Geometry: final body of the model. Coordinates: model frame, mm. A direction names the side the tool comes from. Give positions to 0.01 mm unless a question says otherwise; leave off trailing zeros. Loops run counter-clockwise (first coordinate to the right, second up) from the corner with the lowest first, then second, coordinate; pieces in that order, holes last. Notation, with made-up numbers: (59, 40) - (114, 40) arc R22 ccw to (114, 68) - close; hole circle Ø9 at (23, 13.5). An arc over 180 degrees is marked (long way). Answer in a Markdown table with one row per item.
from build123d import *

# Parameters (mm, degrees)
F0_W      = 76.2
F0_H      = 20.32
F0_R      = 1.905
F1_DEPTH  = 1.524
F2_W      = 50.292
F2_H      = 19.05
F3_DEPTH  = 8.128
F4_W      = 53.467
F4_H      = 35.814
F4_R      = 1.905
F5_DEPTH  = 1.6002
F6_W      = 25.4
F6_H      = 10.16
F7_DEPTH  = 8.128
F8_R      = 1.15
F9_DEPTH  = 3
F11_DEPTH = 3.6
F12_W     = 25
F12_H     = 5
F13_DEPTH = 1.6


with BuildPart() as f1:
    # F0 (on Top) → F1 (new body)
    with BuildSketch(Plane.XY):
        Rectangle(F0_W, F0_H)
        with Locations((-33.02, 0)):
            Circle(F0_R, mode=Mode.SUBTRACT)
        with Locations((33.02, 0)):
            Circle(F0_R, mode=Mode.SUBTRACT)
    extrude(amount=F1_DEPTH)

    # F2 (on face) → F3 (join)
    with BuildSketch(Plane.XY.offset(1.524)):
        Rectangle(F2_W, F2_H)
    extrude(amount=F3_DEPTH)


with BuildPart() as f5:
    # F4 (on Top) → F5 (new body)
    with BuildSketch(Plane.XY):
        with Locations((55.63927, 42.330817)):
            Rectangle(F4_W, F4_H)
        with Locations((33.98577, 40.933817)):
            Circle(F4_R, mode=Mode.SUBTRACT)
        with Locations((72.08577, 40.933817)):
            Circle(F4_R, mode=Mode.SUBTRACT)
    extrude(amount=F5_DEPTH)

    # F6 (on face) → F7 (join)
    with BuildSketch(Plane.XY.offset(1.6002)):
        with Locations((53.03577, 40.933817)):
            Rectangle(F6_W, F6_H)
    extrude(amount=F7_DEPTH)


with BuildPart() as f9:
    # F8 (on Top) → F9 (new body)
    with BuildSketch(Plane.XY):
        with BuildLine():
            ThreePointArc((34.542687, -63.528296), (35.27492, -65.296063), (37.042687, -66.028296))
            Line((37.042687, -66.028296), (97.042687, -66.028296))
            ThreePointArc((97.042687, -66.028296), (98.810454, -65.296063), (99.542687, -63.528296))
            Line((99.542687, -63.528296), (99.542687, -4.528296))
            ThreePointArc((99.542687, -4.528296), (98.810454, -2.760529), (97.042687, -2.028296))
            Line((97.042687, -2.028296), (37.042687, -2.028296))
            ThreePointArc((37.042687, -2.028296), (35.27492, -2.760529), (34.542687, -4.528296))
            Line((34.542687, -4.528296), (34.542687, -63.528296))
        make_face()
        with Locations((37.042687, -63.528296)):
            Circle(F8_R, mode=Mode.SUBTRACT)
        with Locations((97.042687, -63.528296)):
            Circle(F8_R, mode=Mode.SUBTRACT)
        with Locations((37.042687, -4.528296)):
            Circle(F8_R, mode=Mode.SUBTRACT)
        with Locations((97.042687, -4.528296)):
            Circle(F8_R, mode=Mode.SUBTRACT)
    extrude(amount=F9_DEPTH)

    # F10 (on face) → F11 (join)
    with BuildSketch(Plane.XY.offset(3)):
        with BuildLine():
            Line((93.042687, -5.528296), (41.042687, -5.528296))
            ThreePointArc((41.042687, -5.528296), (38.21426, -6.699869), (37.042687, -9.528296))
            Line((37.042687, -9.528296), (37.042687, -58.528296))
            ThreePointArc((37.042687, -58.528296), (38.21426, -61.356723), (41.042687, -62.528296))
            Line((41.042687, -62.528296), (93.042687, -62.528296))
            ThreePointArc((93.042687, -62.528296), (95.871114, -61.356723), (97.042687, -58.528296))
            Line((97.042687, -58.528296), (97.042687, -9.528296))
            ThreePointArc((97.042687, -9.528296), (95.871114, -6.699869), (93.042687, -5.528296))
        make_face()
    extrude(amount=F11_DEPTH)

    # F12 (on face) → F13 (join)
    with BuildSketch(Plane(origin=(0, 0, 0), x_dir=(1, 0, 0), z_dir=(0, 0, -1))):
        with Locations((54.542687, 68.528296)):
            Rectangle(F12_W, F12_H)
        with Locations((79.542687, 68.528296)):
            Rectangle(F12_W, F12_H)
    extrude(amount=-F13_DEPTH)


solid = f1.part
Q1. Cut plane A-A (y = 0). Output: boundary loops of the cut face in (x, z) (3 decimals).
Check values:
| item | result |
|---|---|
| outline | (-38.1, 0) - (-34.925, 0) - (-34.925, 1.524) - (-38.1, 1.524) - close; (-31.115, 0) - (31.115, 0) - (31.115, 1.524) - (25.146, 1.524) - (25.146, 9.652) - (-25.146, 9.652) - (-25.146, 1.524) - (-31.115, 1.524) - close; (34.925, 0) - (38.1, 0) - (38.1, 1.524) - (34.925, 1.524) - close |
Q2. Draft query along Y for faces 4 (the flat face through (0, 9.525, 6)), 5 (the flat face through (-1, -10.16, 1)), 6 (the flat face through (-25.146, 0, 6)), 7 (the cylindrical face through (31.117, 0.084, 0.751)). Return one class per face: pulls with the +Y half, pulls with the -Y half, needs draft (parallel to the pull), parting line crosses it, or undercut.
Check values:
| item | result |
|---|---|
| face 4 | pulls with the +Y half |
| face 5 | pulls with the -Y half |
| face 6 | needs draft |
| face 7 | undercut |
Q3. Cut plane D-D (x = 5.5). Output: boundary loops of the cut face in (y, z) (3 decimals), and give its area (3 significant figures).
Check values:
| item | result |
|---|---|
| outline | (-10.16, 0) - (10.16, 0) - (10.16, 1.524) - (9.525, 1.524) - (9.525, 9.652) - (-9.525, 9.652) - (-9.525, 1.524) - (-10.16, 1.524) - close |
| area | 186 mm² |
Q4. Reachability of faces 1 (the cylindrical face through (-34.923, 0.084, 0.751)), 2 (the flat face through (25.146, 0, 6)), 3 (the flat face through (0, -9.525, 6)) from +Z, -Z, +X, -X, +Y, -Y: full face, straight path, thin tool, end or side. Return the list, or none.
Check values:
| item | result |
|---|---|
| face 1 | +Z, -Z |
| face 2 | +Z, +X, +Y, -Y |
| face 3 | +Z, +X, -X, -Y |
Q5. Cut plane B-B (x = 33.02). Output: boundary loops of the cut face in (y, z) (3 decimals).
Check values:
| item | result |
|---|---|
| outline | (-10.16, 0) - (-1.905, 0) - (-1.905, 1.524) - (-10.16, 1.524) - close; (1.905, 0) - (10.16, 0) - (10.16, 1.524) - (1.905, 1.524) - close |
Q6. Material intervals for line 1 along Y through (x, z) = (-33.02, 1.15) (3 decimals); line 2 along X through (y, z) = (-0.5, 4); line 3 along Y through (x, z) = (-11, 2) (3 decimals), sorted ascending.
Check values:
| item | result |
|---|---|
| line 1 | -10.16 to -1.905, 1.905 to 10.16 |
| line 2 | -25.15 to 25.15 |
| line 3 | -9.525 to 9.525 |
Q7. Cut plane C-C (y = -3.75). Output: boundary loops of the cut face in (x, z).
Check values:
| item | result |
|---|---|
| outline | (-38.1, 0) - (38.1, 0) - (38.1, 1.52) - (25.15, 1.52) - (25.15, 9.65) - (-25.15, 9.65) - (-25.15, 1.52) - (-38.1, 1.52) - close |
Q8. First-contact query: pin 1 (1 mm diameter, centred on y = 2, z = 8, fed in from +X); pin 2 (2.5 mm diameter, centred on x = 9.5, z = 6, fed in from -Y) (3 decimals); pin 3 (5 mm diameter, centred on x = 33.02, y = 0, fed in from +Z). Flat tips, straight axial feed; report the tip coordinate or a pass-through.
Check values:
| item | result |
|---|---|
| pin 1 | x = 25.15 |
| pin 2 | y = -9.525 |
| pin 3 | z = 1.52 |
